```python
from build123d import *

# Parameters (mm, degrees)
F0_W     = 63
F0_H     = 27
F0_W_2   = 55
F0_H_2   = 19
F1_DEPTH = 60
F2_DEPTH = 4
F3_W     = 44
F3_H     = 64
F4_DEPTH = 23
F5_R     = 3.99999
F6_R     = 3


# Not quite as in the source:
# - a fillet or chamfer is up to 0.001 mm smaller than in the source, because OpenCascade refuses the exact size


with BuildPart() as f1:
    # F0 (on Top) → F1 (new body)
    with BuildSketch(Plane.XY):
        Rectangle(F0_W, F0_H)
        Rectangle(F0_W_2, F0_H_2, mode=Mode.SUBTRACT)
    extrude(amount=F1_DEPTH)

    # F0 (on Top) → F2 (join)
    with BuildSketch(Plane.XY):
        Rectangle(F0_W, F0_H)
        Rectangle(F0_W_2, F0_H_2, mode=Mode.SUBTRACT)
        Rectangle(F0_W_2, F0_H_2)
    extrude(amount=-F2_DEPTH)

    # F3 (on face) → F4 (cut)
    with BuildSketch(Plane.XZ.offset(13.5)):
        with Locations((0, 28)):
            Rectangle(F3_W, F3_H)
    extrude(amount=-F4_DEPTH, mode=Mode.SUBTRACT)

    # F5 (radius 4 in the source; OpenCascade refuses exactly that, so slightly less here)
    f5_edges = [f1.edges().sort_by_distance(p)[0] for p in [
        (-22, -11.5, 60),
        (-22, 0, 0),
        (22, 0, 0),
        (-31.5, 0, 60),
        (31.5, 0, 60),
        (22, -11.5, 60),
    ]]
    fillet(f5_edges, radius=F5_R)

    # F6
    f6_edges = [f1.edges().sort_by_distance(p)[0] for p in [
        (-22, -13.5, 26.000005),
        (22, -13.5, 26.000005),
        (23.17157, -13.5, 58.82843),
        (26.75, -13.5, -4),
        (26.75, -13.5, 60),
        (31.5, -13.5, 26.000005),
        (30.32843, -13.5, 58.82843),
    ]]
    fillet(f6_edges, radius=F6_R)


solid = f1.part
```
Here's how the part is built. I have some questions about the finished solid (model axes, mm). A direction names the side the tool comes from. Coordinates: 2 decimals unless noted, no trailing zeros. Order: outer loops, then holes, each group sorted by start corner. A loop starts at its lowest first (then second) coordinate and runs counter-clockwise, first axis right, second up.
1) Imagine slicing it at C-C on x = -15. List the corners of the cut face in (y, z) for me.
2) I need wall thicknesses on line 1 (X direction, y = 4.25, z = 5); line 2 (X direction, y = -10, z = 40); line 3 (Y direction, x = -6, z = 6.5). Which ranges of each line are inside material? Lowest first, please.
3) We'd pull the mould along Y, two halves only. Please class faces 6 (the face through (27, 0, 0)), 7 (the face through (-27.5, 0, 30)), 8 (the face through (27, -13.5, 28)), 9 (the face through (-31.5, 1, 26)): +Y half, -Y half, draft (parallel to the pull), parting line (faces both ways), or undercut.
4) Which directions (+Z, -Z, +X, -X, +Y, -Y) give clear straight access to the entire face, cutting with the end or side of a thin tool? Please do faces 1 (the face through (31.5, 1, 26)), 2 (the face through (-23.203, -9.993, 58.859)), 3 (the face through (-22.86, -12.6, 26.42)), 4 (the face through (-23.203, 0.133, -1.141)), 5 (the face through (26.816, -12.248, -3.438)).
5) Imagine slicing it at B-B on z = 36. List the corners of the cut face in (x, y) for me, and give its area (3 significant figures).
6) Will these pins go through, and if not, where does the flat tip stop? pin 1 (6 mm diameter, centred on x = -3, z = 41.5, fed in from -Y); pin 2 (3 mm diameter, centred on x = 20, y = 0.5, fed in from +Z); pin 3 (1.7 mm diameter, centred on x = -26.5, y = -1, fed in from +Z).
Response values:
1. outline: (9.5, -4) - (13.5, -4) - (13.5, 60) - (9.5, 60) - close
2. line 1: x = -31.5 to -27.5, 27.5 to 31.5
2. line 2: x = -31.5 to -22, 22 to 31.5
2. line 3: y = 9.5 to 13.5
3. face 6: undercut
3. face 7: undercut
3. face 8: -Y half
3. face 9: draft
4. face 1: +Z, -Z, +X, +Y, -Y
4. face 2: +Z, -Y
4. face 3: +Z, -Z, -Y
4. face 4: +Z
4. face 5: -Z, +X, -Y
5. outline: (-31.5, -10.5) arc R3 ccw to (-28.5, -13.5) - (-25, -13.5) arc R3 ccw to (-22, -10.5) - (-22, -9.5) - (-27.5, -9.5) - (-27.5, 9.5) - (27.5, 9.5) - (27.5, -9.5) - (22, -9.5) - (22, -10.5) arc R3 ccw to (25, -13.5) - (28.5, -13.5) arc R3 ccw to (31.5, -10.5) - (31.5, 13.5) - (-31.5, 13.5) - close
5. area: 472 mm2
6. pin 1: stops at y = 9.5
6. pin 2: passes through
6. pin 3: stops at z = 0
